Here's how the part is built. I have some questions about the finished solid (model axes, mm). A direction names the side the tool comes from. Coordinates: 2 decimals unless noted, no trailing zeros. Write each loop counter-clockwise with the first axis right and the second up, starting at its lowest first coordinate (ties: lowest second). Pieces come first, ordered by that corner, then holes.
(1) Imagine slicing it at C-C, the plane x = -14. List the corners of the cut face in (y, z) for me, plus the area to 3 significant figures.
(2) Please list where these lines run through material, in increasing order: probe 1 along X at (y, z) = (-13.25, 3.5); probe 2 along X at (y, z) = (-4, 5.5); probe 3 along X at (y, z) = (-6.5, 2.75).
(3) For pin 1 Ø5 at (x, y) = (14.92, -5.4) entering from +Z; pin 2 Ø3 at (y, z) = (-15, 12.5) entering from -X; pin 3 Ø3 at (y, z) = (-5.5, 8) entering from +X, each with a flat end and sliding along its axis, tell me the tip position at first contact or that it passes through.
(4) Imagine slicing it at B-B, the plane y = -6.25. List the corners of the cut face in (x, z) for me.
(5) Thinking about a two-plate mould opening in Y: for faces 1 (the flat face through (12, -11, 0)), 2 (the flat face through (0, -21.59, 11)), 3 (the cylindrical face through (13.02, -5.31, 2.58)), which applies, released by +Y, released by -Y, zero draft, split by the parting line, or undercut?
(6) Imagine slicing it at A-A, the plane z = 7.75. List the corners of the cut face in (x, y) for me.
(7) Which directions (+Z, -Z, +X, -X, +Y, -Y) give clear straight access to the entire face, cutting with the end or side of a thin tool? Please do faces 4 (the flat face through (15, -11, 5.08)), 5 (the cylindrical face through (-13.16, -16.92, 2.58)), 6 (the flat face through (-15, -11, 5.08)), 7 (the flat face through (6.032, -11, 5)), 8 (the flat face through (0, -11, 15.113)).
(8) Imagine slicing it at D-D, the plane z = 4. List the corners of the cut face in (x, y) for me (1 decimal).
```python
from build123d import *

# Parameters (mm, degrees)
F1_DEPTH = 21.59
F2_R     = 1.905
F3_DEPTH = 5.081


with BuildPart() as f1:
    # F0 (on Front) → F1 (new body)
    with BuildSketch(Plane.XZ):
        Polygon((-18.7325, 5.08), (-18.7325, 0), (-6.0325, 0), (-6.0325, 10.033), (0, 10.033), (6.0325, 10.033), (6.0325, 0), (18.7325, 0), (18.7325, 5.08), (11.1125, 5.08), (11.1125, 15.113), (0, 15.113), (-11.1125, 15.113), (-11.1125, 5.08), align=None)
    extrude(amount=F1_DEPTH)

    # F2 (on face) → F3 (cut, through all)
    with BuildSketch(Plane.XY.offset(5.08)):
        with Locations((-14.9225, -5.3975)):
            Circle(F2_R)
        with Locations((-14.9225, -16.1925)):
            Circle(F2_R)
        with Locations((14.9225, -16.1925)):
            Circle(F2_R)
        with Locations((14.9225, -5.3975)):
            Circle(F2_R)
    extrude(amount=-F3_DEPTH, mode=Mode.SUBTRACT)


solid = f1.part
```
Recorded:
1. outline: (-21.59, 0) - (-17.86, 0) - (-17.86, 5.08) - (-21.59, 5.08) - close; (-14.53, 0) - (-7.06, 0) - (-7.06, 5.08) - (-14.53, 5.08) - close; (-3.73, 0) - (0, 0) - (0, 5.08) - (-3.73, 5.08) - close
1. area: 75.8 mm2
2. probe 1: x = -18.73 to -6.03, 6.03 to 18.73
2. probe 2: x = -11.11 to -6.03, 6.03 to 11.11
2. probe 3: x = -18.73 to -16.48, -13.37 to -6.03, 6.03 to 13.37, 16.48 to 18.73
3. pin 1: stops at z = 5.08
3. pin 2: stops at x = -11.11
3. pin 3: stops at x = 11.11
4. outline: (-18.73, 0) - (-16.63, 0) - (-16.63, 5.08) - (-18.73, 5.08) - close; (-13.22, 0) - (-6.03, 0) - (-6.03, 10.03) - (6.03, 10.03) - (6.03, 0) - (13.22, 0) - (13.22, 5.08) - (11.11, 5.08) - (11.11, 15.11) - (-11.11, 15.11) - (-11.11, 5.08) - (-13.22, 5.08) - close; (16.63, 0) - (18.73, 0) - (18.73, 5.08) - (16.63, 5.08) - close
5. face 1: zero draft
5. face 2: released by -Y
5. face 3: undercut
6. outline: (-11.11, -21.59) - (-6.03, -21.59) - (-6.03, 0) - (-11.11, 0) - close; (6.03, -21.59) - (11.11, -21.59) - (11.11, 0) - (6.03, 0) - close
7. face 4: +Z, +X, +Y, -Y
7. face 5: +Z, -Z
7. face 6: +Z, -X, +Y, -Y
7. face 7: -Z, +Y, -Y
7. face 8: +Z, +X, -X, +Y, -Y
8. outline: (-18.7, -21.6) - (-6, -21.6) - (-6, 0) - (-18.7, 0) - close; (6, -21.6) - (18.7, -21.6) - (18.7, 0) - (6, 0) - close; hole circle Ø3.8 at (-14.9, -16.2); hole circle Ø3.8 at (-14.9, -5.4); hole circle Ø3.8 at (14.9, -16.2); hole circle Ø3.8 at (14.9, -5.4)
